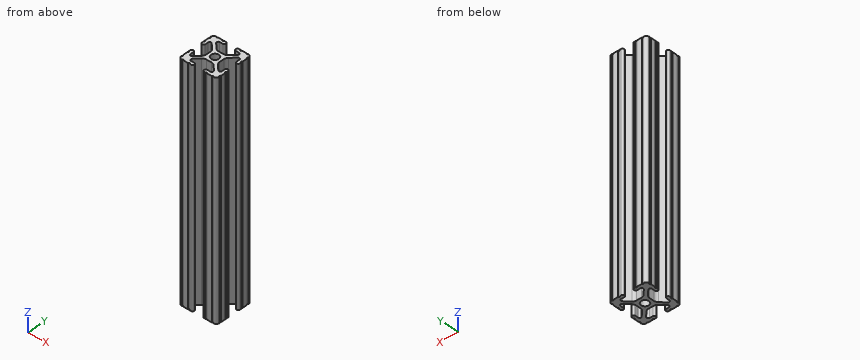
Autodesk Inventor part; units mm, degrees
ref_plane "YZ Plane" through (0, 0, 0) normal (1, 0, 0) x (0, 1, 0)
ref_plane "XZ Plane" through (0, 0, 0) normal (0, 1, 0) x (-1, 0, 0)
ref_plane "XY Plane" through (0, 0, 0) normal (0, 0, 1) x (1, 0, 0)
sketch "Sketch1" plane through (0, 0, 0) normal (0, 0, 1) x (1, 0, 0)
  circle A0 centre (0, 0) radius 2.6035
  arc A1 (-1.7093, -4.4958) -> (-3.9523, -5.4237) centre (-1.7093, -7.6708) ccw
  line L0 (-1.7093, -4.4958) -> (1.7093, -4.4958)
  arc A2 (3.9523, -5.4237) -> (1.7093, -4.4958) centre (1.7093, -7.6708) ccw
  line L1 (3.9523, -5.4237) -> (7.1797, -8.6452)
  arc A3 (6.4164, -10.4902) -> (7.1797, -8.6452) centre (6.4164, -9.4098) ccw
  line L2 (6.4164, -10.4902) -> (4.2875, -10.4902)
  arc A4 (4.2875, -10.4902) -> (3.2385, -11.5392) centre (4.2875, -11.5392) ccw
  line L3 (3.2385, -11.5392) -> (3.2385, -11.651)
  arc A5 (3.2385, -11.651) -> (4.2875, -12.7) centre (4.2875, -11.651) ccw
  line L4 (4.2875, -12.7) -> (5.3171, -12.7)
  arc A6 (6.3331, -12.7) -> (5.3171, -12.7) centre (5.8251, -12.7) ccw
  line L5 (6.3331, -12.7) -> (9.5504, -12.7)
  arc A7 (10.5664, -12.6998) -> (9.5504, -12.7) centre (10.0584, -12.7) ccw
  arc A8 (10.5664, -12.6998) -> (12.6998, -10.5664) centre (10.5918, -10.5918) ccw
  arc A9 (12.7, -9.5504) -> (12.6998, -10.5664) centre (12.7, -10.0584) ccw
  line L6 (12.7, -9.5504) -> (12.7, -6.3331)
  arc A10 (12.7, -5.3171) -> (12.7, -6.3331) centre (12.7, -5.8251) ccw
  line L7 (12.7, -5.3171) -> (12.7, -4.2875)
  arc A11 (12.7, -4.2875) -> (11.651, -3.2385) centre (11.651, -4.2875) ccw
  line L8 (11.651, -3.2385) -> (11.5392, -3.2385)
  arc A12 (11.5392, -3.2385) -> (10.4902, -4.2875) centre (11.5392, -4.2875) ccw
  line L9 (10.4902, -4.2875) -> (10.4902, -6.4021)
  arc A13 (8.7371, -7.1294) -> (10.4902, -6.4021) centre (9.4628, -6.4021) ccw
  line L10 (8.7371, -7.1294) -> (5.441, -3.8408)
  arc A14 (4.5085, -1.5932) -> (5.441, -3.8408) centre (7.6835, -1.5932) ccw
  line L11 (4.5085, -1.5932) -> (4.5085, 1.5932)
  arc A15 (5.441, 3.8408) -> (4.5085, 1.5932) centre (7.6835, 1.5932) ccw
  line L12 (5.441, 3.8408) -> (8.7371, 7.1294)
  arc A16 (10.4902, 6.4021) -> (8.7371, 7.1294) centre (9.4628, 6.4021) ccw
  line L13 (10.4902, 6.4021) -> (10.4902, 4.2875)
  arc A17 (10.4902, 4.2875) -> (11.5392, 3.2385) centre (11.5392, 4.2875) ccw
  line L14 (11.5392, 3.2385) -> (11.651, 3.2385)
  arc A18 (11.651, 3.2385) -> (12.7, 4.2875) centre (11.651, 4.2875) ccw
  line L15 (12.7, 4.2875) -> (12.7, 5.3171)
  arc A19 (12.7, 6.3331) -> (12.7, 5.3171) centre (12.7, 5.8251) ccw
  line L16 (12.7, 6.3331) -> (12.7, 9.5504)
  arc A20 (12.6998, 10.5664) -> (12.7, 9.5504) centre (12.7, 10.0584) ccw
  arc A21 (12.6998, 10.5664) -> (10.5664, 12.6998) centre (10.5918, 10.5918) ccw
  arc A22 (9.5504, 12.7) -> (10.5664, 12.6998) centre (10.0584, 12.7) ccw
  line L17 (9.5504, 12.7) -> (6.3331, 12.7)
  arc A23 (5.3171, 12.7) -> (6.3331, 12.7) centre (5.8251, 12.7) ccw
  line L18 (5.3171, 12.7) -> (4.2875, 12.7)
  arc A24 (4.2875, 12.7) -> (3.2385, 11.651) centre (4.2875, 11.651) ccw
  line L19 (3.2385, 11.651) -> (3.2385, 11.5392)
  arc A25 (3.2385, 11.5392) -> (4.2875, 10.4902) centre (4.2875, 11.5392) ccw
  line L20 (4.2875, 10.4902) -> (6.4768, 10.4902)
  arc A26 (7.207, 8.7244) -> (6.4768, 10.4902) centre (6.4768, 9.4563) ccw
  line L21 (7.207, 8.7244) -> (3.8983, 5.4232)
  arc A27 (1.6558, 4.4958) -> (3.8983, 5.4232) centre (1.6558, 7.6708) ccw
  line L22 (1.6558, 4.4958) -> (-1.6558, 4.4958)
  arc A28 (-3.8983, 5.4232) -> (-1.6558, 4.4958) centre (-1.6558, 7.6708) ccw
  line L23 (-3.8983, 5.4232) -> (-7.207, 8.7244)
  arc A29 (-6.4768, 10.4902) -> (-7.207, 8.7244) centre (-6.4768, 9.4563) ccw
  line L24 (-6.4768, 10.4902) -> (-4.2875, 10.4902)
  arc A30 (-4.2875, 10.4902) -> (-3.2385, 11.5392) centre (-4.2875, 11.5392) ccw
  line L25 (-3.2385, 11.5392) -> (-3.2385, 11.651)
  arc A31 (-3.2385, 11.651) -> (-4.2875, 12.7) centre (-4.2875, 11.651) ccw
  line L26 (-4.2875, 12.7) -> (-5.3171, 12.7)
  arc A32 (-6.3331, 12.7) -> (-5.3171, 12.7) centre (-5.8251, 12.7) ccw
  line L27 (-6.3331, 12.7) -> (-9.5504, 12.7)
  arc A33 (-10.5664, 12.6998) -> (-9.5504, 12.7) centre (-10.0584, 12.7) ccw
  arc A34 (-10.5664, 12.6998) -> (-12.6998, 10.5664) centre (-10.5918, 10.5918) ccw
  arc A35 (-12.7, 9.5504) -> (-12.6998, 10.5664) centre (-12.7, 10.0584) ccw
  line L28 (-12.7, 9.5504) -> (-12.7, 6.3331)
  arc A36 (-12.7, 5.3171) -> (-12.7, 6.3331) centre (-12.7, 5.8251) ccw
  line L29 (-12.7, 5.3171) -> (-12.7, 4.2875)
  arc A37 (-12.7, 4.2875) -> (-11.651, 3.2385) centre (-11.651, 4.2875) ccw
  line L30 (-11.651, 3.2385) -> (-11.5392, 3.2385)
  arc A38 (-11.5392, 3.2385) -> (-10.4902, 4.2875) centre (-11.5392, 4.2875) ccw
  line L31 (-10.4902, 4.2875) -> (-10.4902, 6.4021)
  arc A39 (-8.7371, 7.1294) -> (-10.4902, 6.4021) centre (-9.4628, 6.4021) ccw
  line L32 (-8.7371, 7.1294) -> (-5.441, 3.8408)
  arc A40 (-4.5085, 1.5932) -> (-5.441, 3.8408) centre (-7.6835, 1.5932) ccw
  line L33 (-4.5085, 1.5932) -> (-4.5085, -1.5932)
  arc A41 (-5.441, -3.8408) -> (-4.5085, -1.5932) centre (-7.6835, -1.5932) ccw
  line L34 (-5.441, -3.8408) -> (-8.7371, -7.1294)
  arc A42 (-10.4902, -6.4021) -> (-8.7371, -7.1294) centre (-9.4628, -6.4021) ccw
  line L35 (-10.4902, -6.4021) -> (-10.4902, -4.2875)
  arc A43 (-10.4902, -4.2875) -> (-11.5392, -3.2385) centre (-11.5392, -4.2875) ccw
  line L36 (-11.5392, -3.2385) -> (-11.651, -3.2385)
  arc A44 (-11.651, -3.2385) -> (-12.7, -4.2875) centre (-11.651, -4.2875) ccw
  line L37 (-12.7, -4.2875) -> (-12.7, -5.3171)
  arc A45 (-12.7, -6.3331) -> (-12.7, -5.3171) centre (-12.7, -5.8251) ccw
  line L38 (-12.7, -6.3331) -> (-12.7, -9.5504)
  arc A46 (-12.6998, -10.5664) -> (-12.7, -9.5504) centre (-12.7, -10.0584) ccw
  arc A47 (-12.6998, -10.5664) -> (-10.5664, -12.6998) centre (-10.5918, -10.5918) ccw
  arc A48 (-9.5504, -12.7) -> (-10.5664, -12.6998) centre (-10.0584, -12.7) ccw
  line L39 (-9.5504, -12.7) -> (-6.3331, -12.7)
  arc A49 (-5.3171, -12.7) -> (-6.3331, -12.7) centre (-5.8251, -12.7) ccw
  line L40 (-5.3171, -12.7) -> (-4.2875, -12.7)
  arc A50 (-4.2875, -12.7) -> (-3.2385, -11.651) centre (-4.2875, -11.651) ccw
  line L41 (-3.2385, -11.651) -> (-3.2385, -11.5392)
  arc A51 (-3.2385, -11.5392) -> (-4.2875, -10.4902) centre (-4.2875, -11.5392) ccw
  line L42 (-4.2875, -10.4902) -> (-6.4164, -10.4902)
  arc A52 (-7.1797, -8.6452) -> (-6.4164, -10.4902) centre (-6.4164, -9.4098) ccw
  line L43 (-7.1797, -8.6452) -> (-3.9523, -5.4237)
extrude "Extrusion1" add sketch "Sketch1" against normal blind 152.4
sketch "Sketch2" plane through (0, 0, 0) normal (1, 0, 0) x (0, 1, 0)
  point P0 (0, 0)
properties part number "1010"
Part model, mm, in its own coordinate system. Give positions to 0.01 mm unless a question says otherwise; leave off trailing zeros. Order: outer loops, then holes, each group sorted by start corner. A loop starts at its lowest first (then second) coordinate and runs counter-clockwise, first axis right, second up. Notation, with made-up numbers: M 42.5,27.5 L 57.5,27.5 A17 cw 57.5,43.5 Z; hole C 43,87 d6. An arc over 180 degrees is marked long. Use a Markdown table: item, result. Add a question column.
(1) Drop flat-ended pins along their axis: P1, Ø2, axis at x = 3, z = -34, coming from the -Y side; P2, Ø2, axis at x = -1.5, z = -128.5, coming from the -Y side; P3, Ø1, axis at x = 0, z = -57.5, coming from the +Y side. Give the stop position or say it passes through.
(2) Saw through at A-A, the plane y = 0. Give the cut face in (x, z).
(3) Probe line 1 along X through (y, z) = (-0.25, -101); line 2 along Y through (x, z) = (0, -43.5); line 3 along X through (y, z) = (7, -54). List the from-to ranges inside material, lowest first. Write a range as [from, to].
(4) Saw through at B-B, the plane x = 0. Give the cut face in (y, z), and give its area (3 significant figures).
Answer key:
| question | item | result |
|---|---|---|
| 1 | P1 | y = -12.66 |
| 1 | P2 | y = -4.6 |
| 1 | P3 | y = 4.5 |
| 2 | outline | M -4.51,-152.4 L -2.6,-152.4 L -2.6,0 L -4.51,0 Z; M 2.6,-152.4 L 4.51,-152.4 L 4.51,0 L 2.6,0 Z |
| 3 | line 1 | [-4.51, -2.59], [2.59, 4.51] |
| 3 | line 2 | [-4.5, -2.6], [2.6, 4.5] |
| 3 | line 3 | [-12.7, -10.3], [-8.61, -5.48], [5.48, 8.61], [10.3, 12.7] |
| 4 | outline | M -4.5,-152.4 L -2.6,-152.4 L -2.6,0 L -4.5,0 Z; M 2.6,-152.4 L 4.5,-152.4 L 4.5,0 L 2.6,0 Z |
| 4 | area | 577 mm^2 |
